Design review of the part built by this model. Coordinates are the model's own, in mm. A direction names the side the tool comes from. Coordinates: 2 decimals unless noted, no trailing zeros. Loops run counter-clockwise (first coordinate to the right, second up) from the corner with the lowest first, then second, coordinate; pieces in that order, holes last. Notation, with made-up numbers: (42, -32.75) -> (99, -32.75) arc R7 cw to (99, -23.75) -> close; hole circle Ø3 at (2, 72.5). An arc over 180 degrees is marked (long way). One line per item, written item: value. Start each with the question number.
1. Add section B-B on x = -0.75. Write out the cut boundary in (y, z), plus the area to 3 significant figures.
2. Add section A-A on z = -31. Write out the cut boundary in (x, y).
3. Add section D-D on y = 32.75. Write out the cut boundary in (x, z).
4. Machinability: for faces 1 (the flat face through (-20.926, 46.395, -34.563)), 2 (the flat face through (-6.6, 33, 0)), 3 (the flat face through (-15, 19, -6)), 4 (the flat face through (-16, 39, -2)), which of the approach directions +Z, -Z, +X, -X, +Y, -Y give a long, thin tool a straight path to every point of the face, cutting with its end or side? Answer none if there is none.
5. For probe 1 along Z at (x, y) = (-13.75, 46.5); probe 2 along Z at (x, y) = (-7.75, 51); probe 3 along X at (y, z) = (51.5, -9), list the stretches that pass through material, from the lowest coordinate up.
6. Add section C-C on x = -8.5. Write out the cut boundary in (y, z).
7. Insertion check: pin 1 (8 mm diameter, centred on y = 30, z = -16.5, fed in from -X). The pin has a flat end and moves straight along its axis. Give the tip position at first contact, or say it passes through.
8. Draft analysis for pull direction Z (two halves, no side actions). For faces 5 (the flat face through (-17, 47, -30)), 6 (the flat face through (-4, 33, 3)), 7 (the flat face through (-13, 47, -33)), 8 (the flat face through (1, 54, -18)), state which applies: pulls with the +Z half, pulls with the -Z half, needs draft (parallel to the pull), parting line crosses it, or undercut.
Autodesk Inventor part; units mm, degrees
ref_plane "YZ Plane" through (0, 0, 0) normal (1, 0, 0) x (0, 1, 0)
ref_plane "XZ Plane" through (0, 0, 0) normal (0, 1, 0) x (-1, 0, 0)
ref_plane "XY Plane" through (0, 0, 0) normal (0, 0, 1) x (1, 0, 0)
sketch "Sketch1" plane through (0, 0, 0) normal (0, 0, 1) x (1, 0, 0)
  line L0 (-11.5, 1.5) -> (-11.5, 64)
  line L1 (-1.5, 1.5) -> (-11.5, 1.5)
  line L2 (-1.5, 64) -> (-1.5, 1.5)
  arc A0 (-1.5, 64) -> (-6, 68.5) centre (-6, 64) ccw
  line L3 (-7, 68.5) -> (-6, 68.5)
  arc A1 (-7, 68.5) -> (-11.5, 64) centre (-7, 64) ccw
  line L4 (-13, 64) -> (-13, 1.5)
  line L5 (0, 1.5) -> (0, 64)
  line L6 (-11.5, 0) -> (-1.5, 0)
  arc A2 (-13, 1.5) -> (-11.5, 0) centre (-11.5, 1.5) ccw
  arc A3 (-1.5, 0) -> (0, 1.5) centre (-1.5, 1.5) ccw
  arc A4 (-7, 70) -> (-13, 64) centre (-7, 64) ccw
  arc A5 (0, 64) -> (-6, 70) centre (-6, 64) ccw
  line L7 (-6, 70) -> (-7, 70)
  line L8 (-13, 1.5) -> (-13, 11.5)
  line L9 (-13, 64) -> (-13, 54)
  line L10 (0, 1.5) -> (0, 11.5)
  line L11 (0, 54) -> (0, 64)
  line L12 (0, 11.5) -> (3, 11.5)
  line L13 (3, 11.5) -> (3, 54)
  line L14 (3, 54) -> (0, 54)
  line L15 (0, 11.5) -> (0, 54)
  line L16 (-13, 11.5) -> (-16, 11.5)
  line L17 (-13, 54) -> (-22, 54)
  line L18 (-13, 11.5) -> (-13, 54)
  line L19 (-13, 11.5) -> (-13, 26.5)
  line L20 (-13, 26.5) -> (-18.1176, 26.5)
  line L21 (-13, 54) -> (-13, 39)
  line L22 (-13, 39) -> (-19.8824, 39)
  line L23 (-16, 11.5) -> (-18.1176, 26.5)
  line L24 (-19.8824, 39) -> (-22, 54)
  point P0 (0, 0)
  dimension "d0" = 10
  dimension "d1" = 10
  dimension "d2" = 3
  dimension "d3" = 3
  dimension "d4" = 9
  dimension "d5" = 15
  dimension "d6" = 15
extrude "Extrusion1" add sketch "Sketch1" against normal blind 6 contours L4 L22 L24 L17 | L4 L16 L23 L20 | L14 L13 L12 L5
sketch "Sketch2" plane through (0, 0, 0) normal (0, 0, 1) x (1, 0, 0)
  line L0 (-18.1176, 26.5) -> (-16, 11.5)
  line L1 (-16, 11.5) -> (-13, 11.5)
  line L2 (-13, 26.5) -> (-18.1176, 26.5)
  line L3 (-19.8824, 39) -> (-13, 39)
  line L4 (-22, 54) -> (-19.8824, 39)
  line L5 (-13, 54) -> (-22, 54)
  line L6 (0, 11.5) -> (3, 11.5)
  line L7 (3, 11.5) -> (3, 54)
  line L8 (3, 54) -> (0, 54)
  line L9 (0, 11.5) -> (-13, 11.5)
  line L10 (-13, 54) -> (0, 54)
  arc A0 (-13, 26.5) -> (-13, 39) centre (-13, 32.75) ccw
  point P0 (0, 0)
extrude "Extrusion2" add sketch "Sketch2" along normal blind 3
ref_plane "Work Plane8" through (0, 70, -36) normal (0, 0, -1) x (-1, 0, 0)
sketch "Sketch3" plane through (0, 70, -36) normal (0, 0, -1) x (-1, 0, 0)
  line L0 (22, -16) -> (13, -16)
  line L1 (13, -16) -> (13, -31)
  line L2 (13, -31) -> (19.8824, -31)
  line L3 (19.8824, -31) -> (22, -16)
  line L4 (13, -43.5) -> (13, -58.5)
  line L5 (13, -58.5) -> (16, -58.5)
  line L6 (16, -58.5) -> (18.1176, -43.5)
  line L7 (18.1176, -43.5) -> (13, -43.5)
  line L8 (-3, -58.5) -> (0, -58.5)
  line L9 (0, -58.5) -> (0, -16)
  line L10 (0, -16) -> (-3, -16)
  line L11 (-3, -16) -> (-3, -58.5)
  point P0 (0, -70)
extrude "Extrusion3" add sketch "Sketch3" against normal blind 6
ref_plane "Work Plane7" through (0, 70, -36) normal (0, 0, -1) x (-1, 0, 0)
sketch "Sketch4" plane through (0, 70, -36) normal (0, 0, -1) x (-1, 0, 0)
  line L0 (22, -16) -> (13, -16)
  line L1 (13, -16) -> (13, -31)
  line L2 (13, -31) -> (19.8824, -31)
  line L3 (19.8824, -31) -> (22, -16)
  line L4 (13, -43.5) -> (13, -58.5)
  line L5 (13, -58.5) -> (16, -58.5)
  line L6 (16, -58.5) -> (18.1176, -43.5)
  line L7 (18.1176, -43.5) -> (13, -43.5)
  line L8 (-3, -58.5) -> (0, -58.5)
  line L9 (0, -58.5) -> (0, -16)
  line L10 (0, -16) -> (-3, -16)
  line L11 (-3, -16) -> (-3, -58.5)
  line L12 (18.1176, -43.5) -> (16, -58.5)
  line L13 (16, -58.5) -> (-3, -58.5)
  line L14 (-3, -58.5) -> (-3, -16)
  line L15 (-3, -16) -> (22, -16)
  line L16 (22, -16) -> (19.8824, -31)
  line L17 (19.8824, -31) -> (13, -31)
  arc A0 (13, -31) -> (13, -43.5) centre (13, -37.25) ccw
  line L18 (13, -43.5) -> (18.1176, -43.5)
  point P0 (0, -70)
extrude "Extrusion4" add sketch "Sketch4" along normal blind 3
sketch "Sketch5" plane through (0, 0, -6) normal (0, 0, -1) x (-1, 0, 0)
  line L0 (-3, 11.5) -> (0, 11.5)
  line L1 (0, 11.5) -> (0, 54)
  line L2 (0, 54) -> (-3, 54)
  line L3 (-3, 54) -> (-3, 11.5)
  point P0 (0, 0)
extrude "Extrusion5" add sketch "Sketch5" along normal up to next
properties part number "soporte baterias"
Worked answers:
1. outline: (11.5, -39) -> (54, -39) -> (54, -36) -> (11.5, -36) -> close; (11.5, 0) -> (54, 0) -> (54, 3) -> (11.5, 3) -> close
1. area: 255 mm²
2. outline: (-22, 54) -> (-19.88, 39) -> (-13, 39) -> (-13, 54) -> close; (-18.12, 26.5) -> (-16, 11.5) -> (-13, 11.5) -> (-13, 26.5) -> close; (0, 11.5) -> (3, 11.5) -> (3, 54) -> (0, 54) -> close
3. outline: (-6.75, -39) -> (3, -39) -> (3, 3) -> (-6.75, 3) -> (-6.75, 0) -> (0, 0) -> (0, -36) -> (-6.75, -36) -> close
4. face 1: +Z, -Z, -X, -Y
4. face 2: +Y, -Y
4. face 3: -X, +Y, -Y
4. face 4: +Z, -Z, -X
5. probe 1: z = -39 to -30, -6 to 3
5. probe 2: z = -39 to -36, 0 to 3
5. probe 3: x = 0 to 3
6. outline: (11.5, -39) -> (28.41, -39) -> (28.41, -36) -> (11.5, -36) -> close; (11.5, 0) -> (28.41, 0) -> (28.41, 3) -> (11.5, 3) -> close; (37.09, -39) -> (54, -39) -> (54, -36) -> (37.09, -36) -> close; (37.09, 0) -> (54, 0) -> (54, 3) -> (37.09, 3) -> close
7. pin 1: stops at x = 0
8. face 5: undercut
8. face 6: pulls with the +Z half
8. face 7: undercut
8. face 8: needs draft
